Part model, mm, in its own coordinate system. Face numbers are marked on the shaded views. A direction names the side the tool comes from. Coordinates: 2 decimals unless noted, no trailing zeros. Write each loop counter-clockwise with the first axis right and the second up, starting at its lowest first coordinate (ties: lowest second). Pieces come first, ordered by that corner, then holes. Notation, with made-up numbers: (-6.5, 63.5) -> (36.5, 63.5) arc R24 cw to (36.5, 74.5) -> close; hole circle Ø2 at (-32.75, 29). An arc over 180 degrees is marked (long way). Write item = value, one per line.
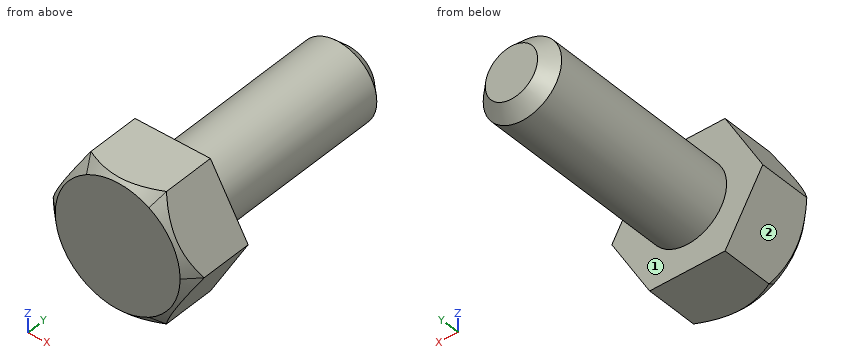
from build123d import *

# Parameters (mm, degrees)
F0_R     = 1.5
F1_DEPTH = 2.5
F2_SIZE  = 0.5
F3_DEPTH = 25
F4_DEPTH = 8
F5_SIZE  = 0.5


with BuildPart() as f1:
    # F0 (on Front) → F1 (new body)
    with BuildSketch(Plane.XZ):
        Polygon((1.443375673, 2.5), (-1.443375673, 2.5), (-2.8867513459, 0), (-1.443375673, -2.5), (1.443375673, -2.5), (2.8867513459, 0), align=None)
        Circle(F0_R, mode=Mode.SUBTRACT)
        Circle(F0_R)
        with BuildLine():
            ThreePointArc((2.8867513459, 0), (2.5, 1.443375673), (1.443375673, 2.5))
            Line((1.443375673, 2.5), (2.8867513459, 0))
        make_face()
        with BuildLine():
            ThreePointArc((1.443375673, 2.5), (0, 2.8867513459), (-1.443375673, 2.5))
            Line((-1.443375673, 2.5), (1.443375673, 2.5))
        make_face()
        with BuildLine():
            Line((1.443375673, -2.5), (-1.443375673, -2.5))
            ThreePointArc((-1.443375673, -2.5), (0, -2.8867513459), (1.443375673, -2.5))
        make_face()
        with BuildLine():
            ThreePointArc((1.443375673, -2.5), (2.5, -1.443375673), (2.8867513459, 0))
            Line((2.8867513459, 0), (1.443375673, -2.5))
        make_face()
        with BuildLine():
            Line((-1.443375673, -2.5), (-2.8867513459, 0))
            ThreePointArc((-2.8867513459, 0), (-2.5, -1.443375673), (-1.443375673, -2.5))
        make_face()
        with BuildLine():
            Line((-2.8867513459, 0), (-1.443375673, 2.5))
            ThreePointArc((-1.443375673, 2.5), (-2.5, 1.443375673), (-2.8867513459, 0))
        make_face()
    extrude(amount=F1_DEPTH)

    # F2
    f2_edges = [f1.edges().sort_by_distance(p)[0] for p in [
        (1.443376, -2.5, -2.5),
    ]]
    chamfer(f2_edges, length=F2_SIZE)

    # F0 (on Front) → F3 (intersect)
    with BuildSketch(Plane.XZ):
        Polygon((1.443375673, 2.5), (-1.443375673, 2.5), (-2.8867513459, 0), (-1.443375673, -2.5), (1.443375673, -2.5), (2.8867513459, 0), align=None)
        Circle(F0_R, mode=Mode.SUBTRACT)
        Circle(F0_R)
    extrude(amount=F3_DEPTH, mode=Mode.INTERSECT)

    # F0 (on Front) → F4 (join)
    with BuildSketch(Plane.XZ):
        Circle(F0_R)
    extrude(amount=-F4_DEPTH)

    # F5
    f5_edges = [f1.edges().sort_by_distance(p)[0] for p in [
        (-1.5, 8, 0),
    ]]
    chamfer(f5_edges, length=F5_SIZE)


solid = f1.part
Q1. Pin check, flat tips, straight feed: pin 1 (1.5 mm diameter, centred on x = -1.5, y = 1.5, fed in from -Z); pin 2 (3 mm diameter, centred on x = 2, y = 6.5, fed in from +Z); pin 3 (1 mm diameter, centred on x = -2.5, y = 3.5, fed in from -Z); pin 4 (1 mm diameter, centred on x = 1.5, y = 2.5, fed in from +Z). Stop position of each tip, or through.
Model answer:
pin_1 = -1.3
pin_2 = 1.41
pin_3 = through
pin_4 = 1.12
Q2. Which spindle directions (+Z, -Z, +X, -X, +Y, -Y) get a long thin tool onto all of the face, cutting with end or side? Do the marked faces 1 and 2. Say none if no direction does.
Model answer:
face_1 = +Y
face_2 = -Z, -X, +Y, -Y
Q3. Saw through at B-B on y = -0.5. Give the cut face in (x, z), and give its area (3 significant figures).
Model answer:
outline = (-2.89, 0) -> (-1.44, -2.5) -> (1.44, -2.5) -> (2.89, 0) -> (1.44, 2.5) -> (-1.44, 2.5) -> close
area = 21.7 mm²
Q4. Probe line 1 (X direction, y = 4, z = -0.4); line 2 (Y direction, x = 1.7, z = 1.05); line 3 (X direction, y = -0.75, z = -2.25). List the from-to ranges inside material, lowest first. Write a range as from..to.
Model answer:
line_1 = -1.45..1.45
line_2 = -2.5..0
line_3 = -1.59..1.59
Q5. Saw through at A-A on x = 0. Give the cut face in (y, z), and give its area (3 significant figures).
Model answer:
outline = (-2.5, -2.39) -> (-2.39, -2.5) -> (0, -2.5) -> (0, -1.5) -> (7.5, -1.5) -> (8, -1) -> (8, 1) -> (7.5, 1.5) -> (0, 1.5) -> (0, 2.5) -> (-2.39, 2.5) -> (-2.5, 2.39) -> close
area = 36.2 mm²
Q6. Saw through at C-C on y = 4.5. Give the cut face in (x, z), and give its area (3 significant figures).
Model answer:
outline = circle Ø3 at (0, 0)
area = 7.07 mm²
